Study the drawing (mm; zero at the part's minimum x, y, z) and answer. A direction names the side the tool comes from. Round coordinates to 2 decimals unless told otherwise and drop trailing zeros. Order: outer loops, then holes, each group sorted by start corner. A loop starts at its lowest first (then second) coordinate and runs counter-clockwise, first axis right, second up. Notation, with made-up numbers: (44, 21) -> (99, 21) arc R16 cw to (99, 37) -> close; hole circle Ø8 at (37, 29.5). An arc over 180 degrees is marked (long way). Answer in a Markdown table with one row per item. Add a question column.
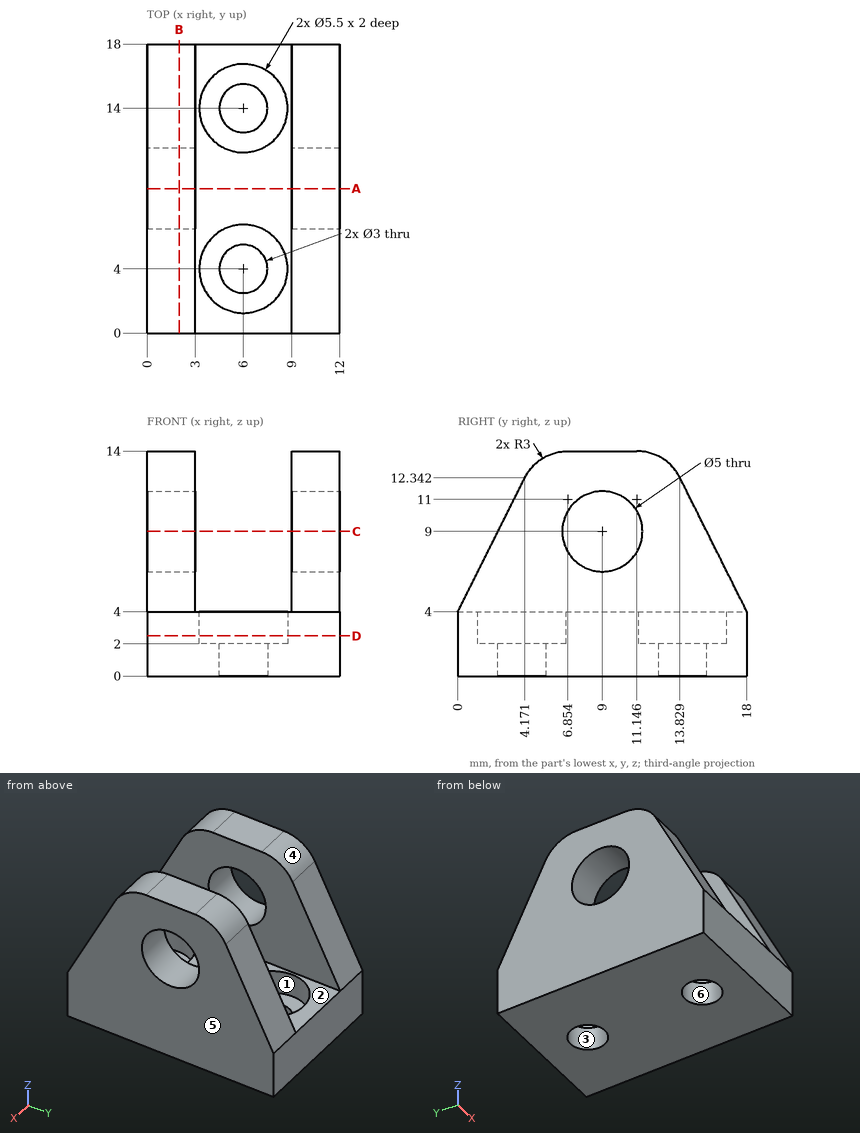
Item 1: The part is cut by section B-B, the plane x = 2. Give the vertices of the cut face in (y, z).
Item 2: Find the intervals of material crossed by probe 1 along Y at (x, z) = (6, 1.05); probe 2 along Z at (x, y) = (1.5, 9); probe 3 along X at (y, z) = (2, 7.75), in increasing order. Write a range as [from, to].
Item 3: For a pull along X with two mould halves and no side action, classify the marked faces 4, 5 and 6 as released by +X, released by -X, zero draft, split by the parting line, or undercut.
Item 4: The part is cut by section C-C, the plane z = 9. Give the vertices of the cut face in (x, y).
Item 5: The part is cut by section A-A, the plane y = 9. Give the vertices of the cut face in (x, z), and give its area (3 significant figures).
Item 6: The part is cut by section D-D, the plane z = 2.5. Give the vertices of the cut face in (x, y).
Item 7: A tool of negligible diameter and unlimited length cuts with its end or side. For the marked faces 1, 2 and 3, from which of +Z, -Z, +X, -X, +Y, -Y can it reach the whole face along a straight path? Write none if from no direction.
Item 8: Flat-ended cylindrical pins translate along their axes: P1, Ø4, axis at x = 6, y = 4, coming from the +Z side; P2, Ø3, axis at x = 7, y = 7.5, coming from the +Z side. Find the tip coordinate at first contact, or state that the pin passes through.
Resolved:
| question | item | result |
|---|---|---|
| 1 | outline | (0, 0) -> (18, 0) -> (18, 4) -> (13.83, 12.34) arc R3 ccw to (11.15, 14) -> (6.85, 14) arc R3 ccw to (4.17, 12.34) -> (0, 4) -> close; hole circle Ø5 at (9, 9) |
| 2 | probe 1 | [0, 2.5], [5.5, 12.5], [15.5, 18] |
| 2 | probe 2 | [0, 6.5], [11.5, 14] |
| 2 | probe 3 | [0, 3], [9, 12] |
| 3 | face 4 | zero draft |
| 3 | face 5 | released by +X |
| 3 | face 6 | undercut |
| 4 | outline | (0, 2.5) -> (3, 2.5) -> (3, 6.5) -> (0, 6.5) -> close; (0, 11.5) -> (3, 11.5) -> (3, 15.5) -> (0, 15.5) -> close; (9, 2.5) -> (12, 2.5) -> (12, 6.5) -> (9, 6.5) -> close; (9, 11.5) -> (12, 11.5) -> (12, 15.5) -> (9, 15.5) -> close |
| 5 | outline | (0, 0) -> (12, 0) -> (12, 6.5) -> (9, 6.5) -> (9, 4) -> (3, 4) -> (3, 6.5) -> (0, 6.5) -> close; (0, 11.5) -> (3, 11.5) -> (3, 14) -> (0, 14) -> close; (9, 11.5) -> (12, 11.5) -> (12, 14) -> (9, 14) -> close |
| 5 | area | 78.0 mm2 |
| 6 | outline | (0, 0) -> (12, 0) -> (12, 18) -> (0, 18) -> close; hole circle Ø5.5 at (6, 4); hole circle Ø5.5 at (6, 14) |
| 7 | face 1 | +Z |
| 7 | face 2 | +Z, +Y, -Y |
| 7 | face 3 | +Z, -Z |
| 8 | P1 | z = 2 |
| 8 | P2 | z = 4 |
